Source: CAD feature listing. Evaluate the final solid. Frame: model axes, mm. A direction names the side the tool comes from. Give positions to 0.01 mm unless a question says otherwise; leave off trailing zeros. Loops run counter-clockwise (first coordinate to the right, second up) from the corner with the lowest first, then second, coordinate; pieces in that order, holes last. Notation, with made-up numbers: M -7,79 L 11,79 A23 ccw 11,114 Z; hole C -10,-20.75 d7. An arc over 180 degrees is marked long. Put each result on its own line as item: value.
from build123d import *

# Parameters (mm, degrees)
BOSS_EXTRUDE1_DEPTH = 4.5
FILLET1_R           = 5
FILLET2_R           = 10
FILLET3_R           = 15


with BuildPart() as part:
    # Sketch1 → Boss-Extrude1 (new body)
    with BuildSketch(Plane.XY):
        Polygon((7.4, 18.5), (28.2, 70.5), (55, 70.5), (55, 75), (30, 75), (40, 100), (100, 100), (100, 0), (100, -5), (0, -5), (0, 0), (-20, 0), align=None)
    extrude(amount=BOSS_EXTRUDE1_DEPTH)

    # Fillet1
    fillet1_edges = [part.edges().sort_by_distance(p)[0] for p in [
        (7.4, 18.5, 2.25),
    ]]
    fillet(fillet1_edges, radius=FILLET1_R)

    # Fillet2
    fillet2_edges = [part.edges().sort_by_distance(p)[0] for p in [
        (100, 100, 2.25),
    ]]
    fillet(fillet2_edges, radius=FILLET2_R)

    # Fillet3
    fillet3_edges = [part.edges().sort_by_distance(p)[0] for p in [
        (40, 100, 2.25),
    ]]
    fillet(fillet3_edges, radius=FILLET3_R)


solid = part.part
1. Contact query for flat-ended pins moving along their axis: P1, Ø12, axis at x = 86.5, y = 59.5, coming from the -Z side; P2, Ø2, axis at x = -10.5, z = 2.5, coming from the -Y side. Output: stop coordinate, or through.
Found:
P1: z = 0
P2: y = 0
2. Section query B-B (x = 13). Output: boundary loops of the cut face in (y, z), plus the area to 3 significant figures.
Found:
outline: M -5,0 L 32.5,0 L 32.5,4.5 L -5,4.5 Z
area: 169 mm^2
3. Section query A-A (z = 0.95). Output: boundary loops of the cut face in (x, y), plus the area to 3 significant figures.
Found:
outline: M -20,0 L 0,0 L 0,-5 L 100,-5 L 100,90 A10 ccw 90,100 L 50.16,100 A15 ccw 36.23,90.57 L 30,75 L 55,75 L 55,70.5 L 28.2,70.5 L 7.97,19.93 A5 cw 6.13,17.64 Z
area: 8,530 mm^2
4. Access query for faces 1 (the flat face through (100, 42, 2)), 2 (the flat face through (0, -3, 2)), 3 (the flat face through (41, 70.5, 2)). Directions: +Z, -Z, +X, -X, +Y, -Y. A direction counts if a zero-diameter tool reaches every point of the face in a straight line with its end or side. Return the directions, or none.
Found:
face 1: +Z, -Z, +X, +Y, -Y
face 2: +Z, -Z, -X, -Y
face 3: +Z, -Z, -X
5. Section query C-C (y = 38.5). Output: boundary loops of the cut face in (x, z), plus the area to 3 significant figures.
Found:
outline: M 15.4,0 L 100,0 L 100,4.5 L 15.4,4.5 Z
area: 381 mm^2
6. Draft query along Y for faces 4 (the flat face through (51, -5, 2)), 5 (the flat face through (55, 73, 2)), 6 (the cylindrical face through (41.85, 97.49, 2.28)). Return one class per face: pulls with the +Y half, pulls with the -Y half, needs draft (parallel to the pull), parting line crosses it, or undercut.
Found:
face 4: pulls with the -Y half
face 5: undercut
face 6: pulls with the +Y half
7. Material intervals for line 1 (Y direction, x = 29, z = 2.75); line 2 (X direction, y = 30, z = 3.6); line 3 (Y direction, x = 93.5, z = 1.6), sorted ascending. Write a range as from..to.
Found:
line 1: -5..70.5
line 2: 12..100
line 3: -5..99.37
